```python
from build123d import *

# Parameters (mm, degrees)
SKETCH2_R           = 1.6637
SKETCH2_R_2         = 0.511037547
SKETCH2_R_3         = 0.469586325
SKETCH2_R_4         = 0.527304242
SKETCH2_R_5         = 0.492462629
SKETCH2_R_6         = 0.523724162
SKETCH2_R_7         = 0.478944742
SKETCH2_R_8         = 0.488742189
SKETCH2_R_9         = 0.503485145
SKETCH2_R_10        = 0.490154406
SKETCH2_R_11        = 0.499999
BOSS_EXTRUDE1_DEPTH = 1.651


with BuildPart() as part:
    # Sketch2 → Boss-Extrude1 (new body)
    with BuildSketch(Plane.XY):
        with BuildLine():
            Line((0, 0), (27.94, 0))
            Line((27.94, 0), (27.94, 13.937675724))
            ThreePointArc((27.94, 13.937675724), (24.7523, 14.605), (27.94, 15.272324276))
            Line((27.94, 15.272324276), (27.94, 34.29))
            Line((27.94, 34.29), (0, 34.29))
            Line((0, 34.29), (0, 15.272324276))
            ThreePointArc((0, 15.272324276), (3.1877, 14.605), (0, 13.937675724))
            Line((0, 13.937675724), (0, 0))
        make_face()
        with Locations(Location((4.445, 22.86, 0), (0, 0, 180))):
            Circle(SKETCH2_R, mode=Mode.SUBTRACT)
        with Locations(Location((4.445, 27.94, 0), (0, 0, 180))):
            Circle(SKETCH2_R, mode=Mode.SUBTRACT)
        with Locations(Location((23.495, 27.94, 0), (0, 0, 180))):
            Circle(SKETCH2_R, mode=Mode.SUBTRACT)
        with Locations((1.905, 7.62)):
            Circle(SKETCH2_R_2, mode=Mode.SUBTRACT)
        with Locations((4.445, 7.62)):
            Circle(SKETCH2_R_3, mode=Mode.SUBTRACT)
        with Locations((6.985, 7.62)):
            Circle(SKETCH2_R_4, mode=Mode.SUBTRACT)
        with Locations((10.16, 7.62)):
            Circle(SKETCH2_R_5, mode=Mode.SUBTRACT)
        with Locations((12.7, 7.62)):
            Circle(SKETCH2_R_6, mode=Mode.SUBTRACT)
        with Locations((15.24, 7.62)):
            Circle(SKETCH2_R_7, mode=Mode.SUBTRACT)
        with Locations((17.78, 7.62)):
            Circle(SKETCH2_R_8, mode=Mode.SUBTRACT)
        with Locations((20.955, 7.62)):
            Circle(SKETCH2_R_9, mode=Mode.SUBTRACT)
        with Locations((23.495, 7.62)):
            Circle(SKETCH2_R_10, mode=Mode.SUBTRACT)
        with Locations((26.035, 7.62)):
            Circle(SKETCH2_R_11, mode=Mode.SUBTRACT)
    extrude(amount=BOSS_EXTRUDE1_DEPTH)


solid = part.part
```
Geometry check sheet. Reference: the model listing, model coordinates, mm. Round coordinates to 2 decimals unless told otherwise and drop trailing zeros. Order: outer loops, then holes, each group sorted by start corner. A loop starts at its lowest first (then second) coordinate and runs counter-clockwise, first axis right, second up. Notation, with made-up numbers: (39.5, 43.5) - (47.5, 43.5) arc R19 cw to (47.5, 67.5) - close; hole circle Ø8 at (14.25, -13.5). An arc over 180 degrees is marked (long way). Use a Markdown table: item, result. Add a question column.
1) Section check C-C (z = 0.4). Count the separate pieces of the cut face and the enclosed holes in it, then the cut area to 3 significant figures.
2) Section check A-A (y = 22.86). Record the cut outline in (x, z), then the cut area to 3 significant figures.
3) Mould release check, pull along X, two halves, no side actions. Record for faces 1 (the flat face through (14, 34.29, 1)), 2 (the cylindrical face through (3.677, 29.416, 0.814)), 3 (the flat face through (0, 7, 1)), 4 (the flat face through (27.94, 7, 1)): released by +X, released by -X, zero draft, split by the parting line, or undercut.
4) Thickness scan on line 1 along Y through (x, z) = (23.5, 0.2); line 2 along Y through (x, z) = (1.5, 1.55); line 3 along X through (y, z) = (28.5, 1.2). Record the ranges inside material, lowest first.
5) Section check B-B (x = 17.78). Record the cut outline in (y, z), then the cut area to 3 significant figures.
6) Section check D-D (x = 23.5). Record the cut outline in (y, z), then the cut area to 3 significant figures.
Established:
| question | item | result |
|---|---|---|
| 1 | separate pieces | 1 |
| 1 | enclosed holes | 13 |
| 1 | area | 907 mm2 |
| 2 | outline | (0, 0) - (2.78, 0) - (2.78, 1.65) - (0, 1.65) - close; (6.11, 0) - (27.94, 0) - (27.94, 1.65) - (6.11, 1.65) - close |
| 2 | area | 40.6 mm2 |
| 3 | face 1 | zero draft |
| 3 | face 2 | undercut |
| 3 | face 3 | released by -X |
| 3 | face 4 | released by +X |
| 4 | line 1 | 0 to 7.13, 8.11 to 26.28, 29.6 to 34.29 |
| 4 | line 2 | 0 to 7.31, 7.93 to 12.94, 16.27 to 34.29 |
| 4 | line 3 | 0 to 2.88, 6.01 to 21.93, 25.06 to 27.94 |
| 5 | outline | (0, 0) - (7.13, 0) - (7.13, 1.65) - (0, 1.65) - close; (8.11, 0) - (34.29, 0) - (34.29, 1.65) - (8.11, 1.65) - close |
| 5 | area | 55.0 mm2 |
| 6 | outline | (0, 0) - (7.13, 0) - (7.13, 1.65) - (0, 1.65) - close; (8.11, 0) - (26.28, 0) - (26.28, 1.65) - (8.11, 1.65) - close; (29.6, 0) - (34.29, 0) - (34.29, 1.65) - (29.6, 1.65) - close |
| 6 | area | 49.5 mm2 |
